CAD build for the part. Positions are in the model's coordinates, mm. A direction names the side the tool comes from. Coordinates: 2 decimals unless noted, no trailing zeros. Write each loop counter-clockwise with the first axis right and the second up, starting at its lowest first coordinate (ties: lowest second). Pieces come first, ordered by that corner, then holes. Notation, with made-up numbers: (33.25, -24.5) - (55.25, -24.5) arc R3 cw to (55.25, -19.5) - close; hole circle Ø6 at (-26.75, 33). An arc over 180 degrees is marked (long way). Answer in a Markdown table with one row per item. Add a question column.
Q1. 3-axis set-ups, long thin cutter, end or side, ignore diameter. For faces 1 (the flat face through (-68.7, -1, 6.2)), 2 (the flat face through (40, 37, -1)), 3 (the flat face through (-48, 1, 0)), 4 (the flat face through (-35, -38, -1)): which of +Z, -Z, +X, -X, +Y, -Y reach the whole face in a straight line?
Q2. Drill centre lines: line 1 along Z through (x, y) = (-48, -59.5); line 2 along X through (y, z) = (-30.5, 5.75); line 3 along Y through (x, z) = (11, 4). Where is each one in solid material? Low to high. Write a range as from..to.
Q3. Band-saw the part on A-A (z = 6). List the corners of the cut face in (x, y), and give its area (3 significant figures).
Q4. Two-plate mould, pull along X, no slides. Class faces 5 (the flat face through (-75, -1, 5)), 6 (the flat face through (46, 1, 0)), 7 (the flat face through (-1, 1, 2.5)): +X half, -X half, draft (parallel to the pull), parting line (faces both ways), or undercut.
Q5. Pin check, flat tips, straight feed: pin 1 (6 mm diameter, centred on x = 28.5, y = 35, fed in from +Z); pin 2 (5 mm diameter, centred on x = 53, y = 39.5, fed in from -Z). Stop position of each tip, or through.
```python
from build123d import *

# Parameters (mm, degrees)
F0_W     = 150
F0_H     = 150
F1_DEPTH = 10
F2_T     = -2.5
F3_SIZE  = 7.49999
F5_DEPTH = 2.5


# Not quite as in the source:
# - a fillet or chamfer is up to 0.001 mm smaller than in the source, because OpenCascade refuses the exact size


with BuildPart() as f1:
    # F0 (on Top) → F1 (new body)
    with BuildSketch(Plane.XY):
        Rectangle(F0_W, F0_H)
    extrude(amount=F1_DEPTH)

    # F2
    f2_openings = [f1.faces().sort_by_distance(p)[0] for p in [
        (0, 0, 10),
    ]]
    offset(amount=F2_T, openings=f2_openings)

    # F3 (size 7.5 in the source; OpenCascade refuses exactly that, so slightly less here)
    f3_edges = [f1.edges().sort_by_distance(p)[0] for p in [
        (-72.5, 0, 2.5),
        (0, 72.5, 2.5),
        (72.5, 0, 2.5),
        (0, -72.5, 2.5),
    ]]
    chamfer(f3_edges, length=F3_SIZE)

    # F4 (on face) → F5 (join)
    with BuildSketch(Plane(origin=(0, 0, 0), x_dir=(1, 0, 0), z_dir=(0, 0, -1))):
        Polygon((0, 3), (-72, 75), (-75, 75), (-75, 72), (-3, 0), (-75, -72), (-75, -75), (-72, -75), (0, -3), (72, -75), (75, -75), (75, -72), (3, 0), (75, 72), (75, 75), (72, 75), align=None)
    extrude(amount=F5_DEPTH)


solid = f1.part
```
Checked values:
| question | item | result |
|---|---|---|
| 1 | face 1 | +Z |
| 1 | face 2 | -Z, +X |
| 1 | face 3 | -Z, -X |
| 1 | face 4 | -Z, -Y |
| 2 | line 1 | z = 0..2.5 |
| 2 | line 2 | x = -75..-68.25, 68.25..75 |
| 2 | line 3 | y = -75..-66.5, 66.5..75 |
| 3 | outline | (-75, -75) - (75, -75) - (75, 75) - (-75, 75) - close; hole (-68.5, -68.5) - (68.5, -68.5) - (68.5, 68.5) - (-68.5, 68.5) - close |
| 3 | area | 3,730 mm² |
| 4 | face 5 | -X half |
| 4 | face 6 | draft |
| 4 | face 7 | undercut |
| 5 | pin 1 | stops at z = 2.5 |
| 5 | pin 2 | stops at z = 0 |
